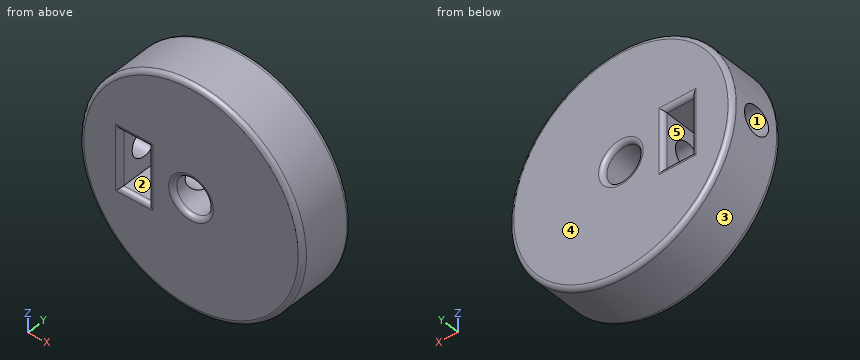
```python
from build123d import *

# Parameters (mm, degrees)
SKETCH1_R                      = 25
SKETCH1_R_2                    = 4
BOSS_EXTRUDE1_DEPTH            = 12.7
SKETCH2_W                      = 6.35
SKETCH2_H                      = 12.7
CUT_EXTRUDE1_DEPTH             = 38.567139896
SKETCH3_R                      = 3.175
CUT_EXTRUDE2_DEPTH             = 45.477698063
CUT_EXTRUDE2_DIRECTION_2_REACH = 46.478
FILLET1_R                      = 1


with BuildPart() as part:
    # Sketch1 → Boss-Extrude1 (new body)
    with BuildSketch(Plane(origin=(0, 0, 0), x_dir=(1, 0, 0), z_dir=(0, 1, 0))):
        with Locations(Location((0, 0, 0), (0, 0, 270))):
            Circle(SKETCH1_R)
        with Locations(Location((0, 0, 0), (0, 0, 270))):
            Circle(SKETCH1_R_2, mode=Mode.SUBTRACT)
    extrude(amount=BOSS_EXTRUDE1_DEPTH)

    # Sketch2 → Cut-Extrude1 (cut, through all)
    with BuildSketch(Plane(origin=(0, 12.7, 0), x_dir=(1, 0, 0), z_dir=(0, 1, 0))):
        with Locations((-12.7, 0)):
            Rectangle(SKETCH2_W, SKETCH2_H)
    extrude(amount=-CUT_EXTRUDE1_DEPTH, mode=Mode.SUBTRACT)

    # Sketch3 → Cut-Extrude2 (cut)
    with BuildSketch(Plane.ZY.offset(9.525)):
        with Locations((0, 6.35)):
            Circle(SKETCH3_R)
    extrude(amount=CUT_EXTRUDE2_DEPTH, mode=Mode.SUBTRACT)

    # Sketch3 → Cut-Extrude2 direction 2 (cut, up to next)
    with BuildSketch(Plane.ZY.offset(9.525), mode=Mode.PRIVATE) as cut_extrude2_direction_2_sk1:
        with Locations((0, 6.35)):
            Circle(SKETCH3_R)
    cut_extrude2_direction_2_tool1 = extrude(cut_extrude2_direction_2_sk1.sketch, amount=-CUT_EXTRUDE2_DIRECTION_2_REACH, mode=Mode.PRIVATE) & part.part
    add(cut_extrude2_direction_2_tool1.solids().sort_by_distance((-9.525, 6.35, 0))[0], mode=Mode.SUBTRACT)

    # Fillet1
    fillet1_edges = [part.edges().sort_by_distance(p)[0] for p in [
        (-15.875, 0, 0),
        (-12.7, 0, -6.35),
        (-9.525, 0, 0),
        (-12.7, 0, 6.35),
        (-15.875, 12.7, 0),
        (-12.7, 12.7, 6.35),
        (-9.525, 12.7, 0),
        (-12.7, 12.7, -6.35),
        (0, 0, -25),
        (0, 12.7, -25),
        (0, 0, -4),
        (0, 12.7, -4),
    ]]
    fillet(fillet1_edges, radius=FILLET1_R)


solid = part.part
```
CAD build for the part. Positions are in the model's coordinates, mm. Face numbers are marked on the shaded views. A direction names the side the tool comes from. Round coordinates to 2 decimals unless told otherwise and drop trailing zeros. Order: outer loops, then holes, each group sorted by start corner. A loop starts at its lowest first (then second) coordinate and runs counter-clockwise, first axis right, second up. Notation, with made-up numbers: (7.5, 75.25) -> (43.5, 75.25) arc R13 cw to (43.5, 83.25) -> close; hole circle Ø6 at (58.5, 45). An arc over 180 degrees is marked (long way). One line per question, with ' | ' between items.
Q1. Slice it at A-A (z = 0). Give the number of separate pieces and of enclosed holes in the cut face, then the cut area to 3 significant figures.
Completed:
separate pieces: 5 | enclosed holes: 0 | area: 357 mm^2
Q2. Slice it at D-D (y = 6.35). Write the cut outline in (x, z) (3 decimals), then the cut area to 3 significant figures.
Completed:
outline: (-24.798, -3.175) arc R25 ccw (long way) to (-24.798, 3.175) -> (-15.875, 3.175) -> (-15.875, 6.35) -> (-9.525, 6.35) -> (-9.525, 3.175) -> (-2.433, 3.175) arc R4 cw (long way) to (-2.433, -3.175) -> (-9.525, -3.175) -> (-9.525, -6.35) -> (-15.875, -6.35) -> (-15.875, -3.175) -> close | area: 1,740 mm^2
Q3. Slice it at C-C (y = 2.25). Write the cut outline in (x, z) (3 decimals).
Completed:
outline: circle Ø50 at (0, 0); hole (-15.875, -6.35) -> (-9.525, -6.35) -> (-9.525, 6.35) -> (-15.875, 6.35) -> close; hole circle Ø8 at (0, 0)
Q4. Which spindle directions (+Z, -Z, +X, -X, +Y, -Y) get a long thin tool onto all of the face, cutting with end or side? Do the marked faces 4 and 5. Say none if no direction does.
Completed:
face 4: +Z, -Z, +X, -X, +Y | face 5: +Y, -Y
Q5. Drop flat-ended pins along their axis: pin 1 (6 mm diameter, centred on x = 15.5, y = 9, fed in from -Z); pin 2 (3 mm diameter, centred on x = 15.5, y = 9, fed in from -Z); pin 3 (4 mm diameter, centred on y = 6.35, z = 0, fed in from -X). Give the stop position or say it passes through.
Completed:
pin 1: stops at z = -21.65 | pin 2: stops at z = -20.71 | pin 3: stops at x = 3.46
Q6. Probe probe 1 along Y at (x, z) = (-20, 0) (3 decimals); probe 2 along X at (y, z) = (9.75, 1.5) (3 decimals); probe 3 along X at (y, z) = (9.5, -3.5) (1 decimal). List the from-to ranges inside material, lowest first.
Completed:
probe 1: y = 0 to 3.175, 9.525 to 12.7 | probe 2: x = -24.955 to -15.875, -9.525 to -3.708, 3.708 to 24.955 | probe 3: x = -24.8 to -15.9, -9.5 to -1.9, 1.9 to 24.8
Q7. Slice it at B-B (x = 0). Write the cut outline in (y, z).
Completed:
outline: (0, -24) arc R1 ccw to (1, -25) -> (11.7, -25) arc R1 ccw to (12.7, -24) -> (12.7, -5) arc R1 ccw to (11.7, -4) -> (1, -4) arc R1 ccw to (0, -5) -> close; (0, 5) arc R1 ccw to (1, 4) -> (11.7, 4) arc R1 ccw to (12.7, 5) -> (12.7, 24) arc R1 ccw to (11.7, 25) -> (1, 25) arc R1 ccw to (0, 24) -> close
Q8. Two-plate mould, pull along X, no slides. Class the marked faces 1, 2 and 3: released by +X, released by -X, zero draft, split by the parting line, or undercut.
Completed:
face 1: zero draft | face 2: undercut | face 3: split by the parting line
